from build123d import *

# Parameters (mm, degrees)
SKETCH_1_W          = 65
SKETCH_1_H          = 68
SKETCH_1_R          = 21
EXTRUDE_1_DEPTH     = 6
SKETCH_3_W          = 62
SKETCH_3_H          = 6
EXTRUDE_2_DEPTH     = 65
CHAMFER_2_SIZE      = 6
CHAMFER_3_SIZE      = 6
CHAMFER_4_SIZE      = 6
CHAMFER_5_SIZE      = 6
FILLET_1_R          = 2
FILLET_2_R          = 2
SKETCH_5_R          = 2.75
CUT_EXTRUDE_3_DEPTH = 88.759227349
SKETCH_6_R          = 2.75
CUT_EXTRUDE_4_DEPTH = 95.80177845


with BuildPart() as part:
    # Sketch 1 → Extrude 1 (new body)
    with BuildSketch(Plane.XY):
        with Locations((3.546875, 16.5796875)):
            Rectangle(SKETCH_1_W, SKETCH_1_H)
        with Locations((3.546875, 21.5796875)):
            Circle(SKETCH_1_R, mode=Mode.SUBTRACT)
    extrude(amount=EXTRUDE_1_DEPTH)

    # Sketch 3 → Extrude 2 (add)
    with BuildSketch(Plane(origin=(36.046875, 0, 0), x_dir=(0, 0, -1), z_dir=(1, 0, 0))):
        with Locations((31, -14.4203125)):
            Rectangle(SKETCH_3_W, SKETCH_3_H)
    extrude(amount=-EXTRUDE_2_DEPTH)

    # Chamfer 2
    chamfer_2_edges = [part.edges().sort_by_distance(p)[0] for p in [
        (36.046875, -14.4203125, -62),
    ]]
    chamfer(chamfer_2_edges, length=CHAMFER_2_SIZE)

    # Chamfer 3
    chamfer_3_edges = [part.edges().sort_by_distance(p)[0] for p in [
        (-28.953125, -14.4203125, -62),
    ]]
    chamfer(chamfer_3_edges, length=CHAMFER_3_SIZE)

    # Chamfer 4
    chamfer_4_edges = [part.edges().sort_by_distance(p)[0] for p in [
        (-28.953125, 50.5796875, 3),
    ]]
    chamfer(chamfer_4_edges, length=CHAMFER_4_SIZE)

    # Chamfer 5
    chamfer_5_edges = [part.edges().sort_by_distance(p)[0] for p in [
        (36.046875, 50.5796875, 3),
    ]]
    chamfer(chamfer_5_edges, length=CHAMFER_5_SIZE)

    # Fillet 1
    fillet_1_edges = [part.edges().sort_by_distance(p)[0] for p in [
        (3.546875, -17.4203125, 6),
    ]]
    fillet(fillet_1_edges, radius=FILLET_1_R)

    # Fillet 2
    fillet_2_edges = [part.edges().sort_by_distance(p)[0] for p in [
        (3.546875, -11.4203125, 0),
    ]]
    fillet(fillet_2_edges, radius=FILLET_2_R)

    # Sketch 5 → Cut-Extrude 3 (cut, through all)
    with BuildSketch(Plane(origin=(0, 0, 0), x_dir=(-1, 0, 0), z_dir=(0, 0, -1))):
        with Locations((-27.046875, 45.0796875)):
            Circle(SKETCH_5_R)
        with Locations(Location((19.953125, 45.0796875, 0), (0, 0, 180))):
            Circle(SKETCH_5_R)
        with Locations((19.953125, -1.9203125)):
            Circle(SKETCH_5_R)
        with Locations(Location((-27.046875, -1.9203125, 0), (0, 0, 180))):
            Circle(SKETCH_5_R)
    extrude(amount=-CUT_EXTRUDE_3_DEPTH, mode=Mode.SUBTRACT)

    # Sketch 6 → Cut-Extrude 4 (cut, through all)
    with BuildSketch(Plane(origin=(0, -11.4203125, 0), x_dir=(1, 0, 0), z_dir=(0, 1, 0))):
        with Locations(Location((23.546875, 11.156752463, 0), (0, 0, 180))):
            Circle(SKETCH_6_R)
        with Locations(Location((23.546875, 53.156752463, 0), (0, 0, 180))):
            Circle(SKETCH_6_R)
        with Locations((-16.453125, 53.156752463)):
            Circle(SKETCH_6_R)
        with Locations((-16.453125, 11.156752463)):
            Circle(SKETCH_6_R)
    extrude(amount=-CUT_EXTRUDE_4_DEPTH, mode=Mode.SUBTRACT)


solid = part.part
CAD build for the part. Positions are in the model's coordinates, mm. A direction names the side the tool comes from. Coordinates: 2 decimals unless noted, no trailing zeros. Loops run counter-clockwise (first coordinate to the right, second up) from the corner with the lowest first, then second, coordinate; pieces in that order, holes last. Notation, with made-up numbers: (40.5, -6.75) - (95.5, -6.75) arc R24 cw to (95.5, 30.25) - close; hole circle Ø10 at (1.5, -26.75). An arc over 180 degrees is marked (long way). Use one line per item in the form item = value. Start each with the question number.
1) Band-saw the part on C-C (x = 28). Give the cut face in (y, z).
2) Drill centre lines: L1, parallel to Y at x = -7.5, z = -49; L2, parallel to Z at x = 25, y = 11. Where is each one in solid material? Low to high. Write a range as from..to.
3) Band-saw the part on A-A (y = 7.5). Give the cut face in (x, z), and give its area (3 significant figures).
4) Band-saw the part on B-B (x = -1.5). Give the cut face in (y, z).
5) Tool access for faces 1 (the face through (4, -11.42, -32)), 2 (the face through (-22.7, 45, 3)): list every direction of +Z, -Z, +X, -X, +Y, -Y with a clear straight run to the whole face (end or side of a thin tool).
6) Flat gauge pins, fed straight in: pin 1 (1.5 mm diameter, centred on x = 28.5, z = -27.5, fed in from +Y); pin 2 (6 mm diameter, centred on x = 13.5, y = -5.5, fed in from -Z). Where does each tip first touch, or does it go through?
7) Two-plate mould, pull along Y, no slides. Class faces 3 (the face through (-17.206, -1.799, 2.958)), 4 (the face through (18, 3, 6)), 5 (the face through (4, -16.82, 5.43)): +Y half, -Y half, draft (parallel to the pull), parting line (faces both ways), or undercut.
8) Band-saw the part on D-D (y = 20.5). Give the cut face in (x, z).
Check values:
q1.outline = (-17.42, -62) - (-11.42, -62) - (-11.42, -2) arc R2 cw to (-9.42, 0) - (-4.5, 0) - (-4.5, 6) - (-15.42, 6) arc R2 ccw to (-17.42, 4) - close; (0.66, 0) - (42.5, 0) - (42.5, 6) - (0.66, 6) - close; (47.66, 0) - (50.58, 0) - (50.58, 6) - (47.66, 6) - close
q2.L1 = -17.42..-11.42
q2.L2 = 0..6
q3.outline = (-28.95, 0) - (-12.03, 0) - (-12.03, 6) - (-28.95, 6) - close; (19.13, 0) - (36.05, 0) - (36.05, 6) - (19.13, 6) - close
q3.area = 203 mm2
q4.outline = (-17.42, -62) - (-11.42, -62) - (-11.42, -2) arc R2 cw to (-9.42, 0) - (1.2, 0) - (1.2, 6) - (-15.42, 6) arc R2 ccw to (-17.42, 4) - close; (41.96, 0) - (50.58, 0) - (50.58, 6) - (41.96, 6) - close
q5.face_1 = -Z, +X, -X, +Y
q5.face_2 = +Z, -Z
q6.pin_1 = -11.42
q6.pin_2 = 0
q7.face_3 = undercut
q7.face_4 = draft
q7.face_5 = -Y half
q8.outline = (-28.95, 0) - (-17.43, 0) - (-17.43, 6) - (-28.95, 6) - close; (24.52, 0) - (36.05, 0) - (36.05, 6) - (24.52, 6) - close
